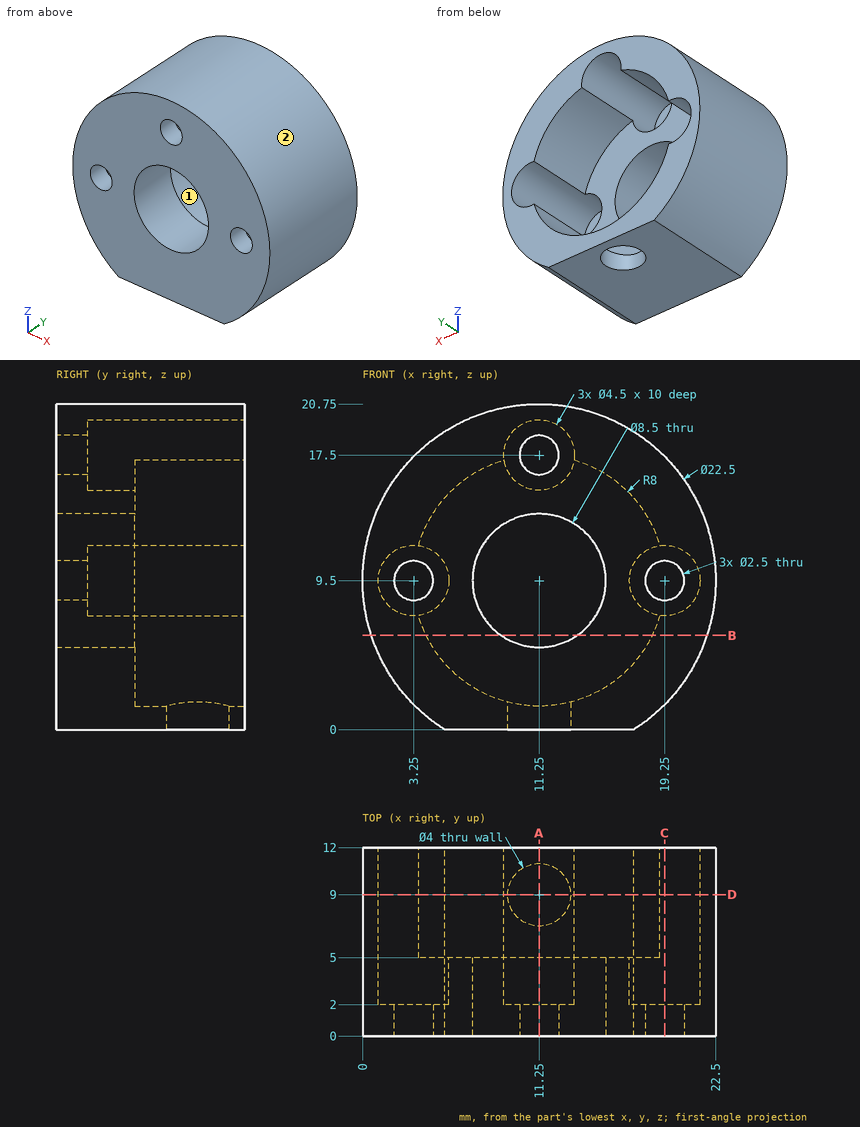
For this review, use the dimensioned drawing (mm, ordinates from the lowest corner) and the shaded views. A direction names the side the tool comes from. Round coordinates to 2 decimals unless told otherwise and drop trailing zeros. Order: outer loops, then holes, each group sorted by start corner. A loop starts at its lowest first (then second) coordinate and runs counter-clockwise, first axis right, second up. Notation, with made-up numbers: (28.25, 51.5) -> (79.25, 51.5) arc R10 ccw to (79.25, 70.5) -> close; hole circle Ø9 at (37, 5.5). An arc over 180 degrees is marked (long way). One line per item, written item: value. Start each with the question number.
Q1. Machinability: for the marked faces 1 and 2, which of the approach directions +Z, -Z, +X, -X, +Y, -Y give a long, thin tool a straight path to every point of the face, cutting with its end or side? Answer none if there is none.
Q2. Clearance check with flat-ended pins moving along their axes: pin 1 Ø1.3 at (x, z) = (2.5, 10.5) entering from +Y; pin 2 Ø6 at (y, z) = (4.5, 2) entering from -X; pin 3 Ø7.5 at (x, z) = (13, 11.5) entering from +Y; pin 4 Ø2 at (x, z) = (3.25, 9.5) entering from -Y. State where each tip first meets the part, or that it passes through.
Q3. Take a section at D-D (y = 9). Write out the cut boundary in (x, z), and give its area (3 significant figures).
Q4. Take a section at B-B (z = 6). Write out the cut boundary in (x, y).
Q5. Take a section at A-A (x = 11.25). Write out the cut boundary in (y, z).
Q6. Wall thickness on line 1 (Z direction, x = 12, y = 4.75); line 2 (X direction, y = 7.25, z = 11); line 3 (X direction, y = 9.5, z = 6): over which ranges is each line inside the solid? List them lowest first.
Q7. Take a section at C-C (x = 19.25). Write out the cut boundary in (y, z).
Reported:
1. face 1: +Y
1. face 2: +Y, -Y
2. pin 1: stops at y = 2
2. pin 2: stops at x = 0.94
2. pin 3: stops at y = 5
2. pin 4: passes through
3. outline: (3.57, 7.27) arc R2.25 cw (long way) to (3.57, 11.73) arc R8 cw to (9.02, 17.18) arc R2.25 cw (long way) to (13.48, 17.18) arc R8 cw to (18.93, 11.73) arc R2.25 cw (long way) to (18.93, 7.27) arc R8 cw to (13.25, 1.75) -> (13.25, 0) -> (17.28, 0) arc R11.25 ccw (long way) to (5.22, 0) -> (9.25, 0) -> (9.25, 1.75) arc R8 cw to start
3. area: 151 mm2
4. outline: (0.56, 0) -> (8.84, 0) -> (8.84, 5) -> (4.06, 5) -> (4.06, 12) -> (0.56, 12) -> close; (13.66, 0) -> (21.94, 0) -> (21.94, 12) -> (18.44, 12) -> (18.44, 5) -> (13.66, 5) -> close
5. outline: (0, 0) -> (7, 0) -> (7, 1.5) -> (5, 1.5) -> (5, 5.25) -> (0, 5.25) -> close; (0, 13.75) -> (5, 13.75) -> (5, 15.25) -> (2, 15.25) -> (2, 16.25) -> (0, 16.25) -> close; (0, 18.75) -> (2, 18.75) -> (2, 19.75) -> (12, 19.75) -> (12, 20.75) -> (0, 20.75) -> close; (11, 0) -> (12, 0) -> (12, 1.5) -> (11, 1.5) -> close
6. line 1: z = 0 to 5.32, 13.68 to 15.38, 19.62 to 20.72
6. line 2: x = 0.1 to 1.57, 20.93 to 22.4
6. line 3: x = 0.56 to 4.06, 18.44 to 21.94
7. outline: (0, 1.59) -> (12, 1.59) -> (12, 7.25) -> (2, 7.25) -> (2, 8.25) -> (0, 8.25) -> close; (0, 10.75) -> (2, 10.75) -> (2, 11.75) -> (12, 11.75) -> (12, 17.41) -> (0, 17.41) -> close
